```python
from build123d import *

# Parameters (mm, degrees)
SKETCH1_W           = 10
SKETCH1_H           = 4
BOSS_EXTRUDE1_DEPTH = 9
CUT_EXTRUDE1_DEPTH  = 5
SKETCH3_R           = 0.3
BOSS_EXTRUDE2_DEPTH = 1
FILLET1_R           = 0.2


with BuildPart() as part:
    # Sketch1 → Boss-Extrude1 (new body)
    with BuildSketch(Plane(origin=(0, 0, 0), x_dir=(1, 0, 0), z_dir=(0, 1, 0))):
        Rectangle(SKETCH1_W, SKETCH1_H)
    extrude(amount=BOSS_EXTRUDE1_DEPTH)

    # Sketch2 → Cut-Extrude1 (cut, through all)
    with BuildSketch(Plane.XY.offset(2)):
        Polygon((-3, 0), (-2.5, 0.5), (2.5, 0.5), (3, 0), (3, -1.5), (-3, -1.5), align=None)
    extrude(amount=-CUT_EXTRUDE1_DEPTH, mode=Mode.SUBTRACT)

    # Sketch3 → Boss-Extrude2 (add)
    with BuildSketch(Plane.XZ):
        with Locations((3.75, 0)):
            Circle(SKETCH3_R)
        with Locations((-3.75, 0)):
            Circle(SKETCH3_R)
    extrude(amount=BOSS_EXTRUDE2_DEPTH)

    # Fillet1
    fillet1_edges = [part.edges().sort_by_distance(p)[0] for p in [
        (5, 9, 0),
        (0, 9, -2),
        (-4, 0, -2),
        (4, 0, 2),
        (2.75, 0.25, 2),
        (0, 0.5, 2),
        (-2.75, 0.25, 2),
        (-2.75, 0.25, -2),
        (-3, 0, 0),
        (0, 0.5, -2),
        (-2.5, 0.5, 0),
        (2.75, 0.25, -2),
        (2.5, 0.5, 0),
        (3, 0, 0),
        (-5, 9, 0),
        (4, 0, -2),
        (5, 0, 0),
        (-4, 0, 2),
        (-5, 0, 0),
        (0, 9, 2),
        (-5, 4.5, -2),
        (5, 4.5, -2),
        (5, 4.5, 2),
        (-5, 4.5, 2),
    ]]
    fillet(fillet1_edges, radius=FILLET1_R)


solid = part.part
```
Could you check a few things on this model? Use its own coordinates, in mm. Round coordinates to 2 decimals unless told otherwise and drop trailing zeros. Write each loop counter-clockwise with the first axis right and the second up, starting at its lowest first coordinate (ties: lowest second). Pieces come first, ordered by that corner, then holes.
(1) If I drill on probe 1 along Y at (x, z) = (-4, -1.65); probe 2 along Y at (x, z) = (1.25, 0.25); probe 3 along X at (y, z) = (4.25, 1.85), over which ranges is the centre line in solid material (lowest first)?
Findings below:
probe 1: y = 0 to 9
probe 2: y = 0.5 to 9
probe 3: x = -4.99 to 4.99
(2) Suppose I cut it at C-C on x = -3.75. Write out the boundary of the cut face in (y, z), and give its area (3 significant figures).
Findings below:
outline: (-1, -0.3) - (0, -0.3) - (0, -1.8) arc R0.2 ccw to (0.2, -2) - (8.8, -2) arc R0.2 ccw to (9, -1.8) - (9, 1.8) arc R0.2 ccw to (8.8, 2) - (0.2, 2) arc R0.2 ccw to (0, 1.8) - (0, 0.3) - (-1, 0.3) - close
area: 36.6 mm2
(3) Suppose I cut it at B-B on z = -0.45. Write out the boundary of the cut face in (x, y).
Findings below:
outline: (-5, 0.2) arc R0.2 ccw to (-4.8, 0) - (-3.08, 0) arc R0.2 ccw to (-2.94, 0.06) - (-2.56, 0.44) arc R0.2 cw to (-2.42, 0.5) - (2.42, 0.5) arc R0.2 cw to (2.56, 0.44) - (2.94, 0.06) arc R0.2 ccw to (3.08, 0) - (4.8, 0) arc R0.2 ccw to (5, 0.2) - (5, 8.8) arc R0.2 ccw to (4.8, 9) - (-4.8, 9) arc R0.2 ccw to (-5, 8.8) - close
(4) For pin 1 (1.4 mm diameter, centred on x = 4, z = -0.5, fed in from -Y); pin 2 (1.8 mm diameter, centred on x = 1, z = 0, fed in from -Y), each with a flat end and sliding along its axis, tell me the tip position at first contact or that it passes through.
Findings below:
pin 1: stops at y = -1
pin 2: stops at y = 0.5
(5) Suppose I cut it at D-D on x = 4.25. Write out the boundary of the cut face in (y, z), and give its area (3 significant figures).
Findings below:
outline: (0, -1.8) arc R0.2 ccw to (0.2, -2) - (8.8, -2) arc R0.2 ccw to (9, -1.8) - (9, 1.8) arc R0.2 ccw to (8.8, 2) - (0.2, 2) arc R0.2 ccw to (0, 1.8) - close
area: 36.0 mm2
(6) Thinking about a two-plate mould opening in X: for faces 1 (the face through (0, 0.5, 0)), 2 (the face through (5, 4, 0)), 3 (the face through (0, 4, -2)), which applies, +X half, -X half, draft (parallel to the pull), parting line (faces both ways), or undercut?
Findings below:
face 1: undercut
face 2: +X half
face 3: draft
(7) Suppose I cut it at A-A on x = -1.75. Write out the boundary of the cut face in (y, z).
Findings below:
outline: (0.5, -1.8) arc R0.2 ccw to (0.7, -2) - (8.8, -2) arc R0.2 ccw to (9, -1.8) - (9, 1.8) arc R0.2 ccw to (8.8, 2) - (0.7, 2) arc R0.2 ccw to (0.5, 1.8) - close
